```python
from build123d import *

# Parameters (mm, degrees)
EXTRUDE_1_DEPTH      = 13.8
EXTRUDE_1_DEPTH_BACK = 13.8
EXTRUDE_START        = -2
SKETCH_2_W           = 14
SKETCH_2_H           = 6
SKETCH_2_W_2         = 10
SKETCH_2_H_2         = 2
EXTRUDE_2_DEPTH      = 2
EXTRUDE_3_DEPTH      = 1
EXTRUDE_3_DEPTH_BACK = 3
SKETCH_3_R           = 3
EXTRUDE_4_DEPTH      = 3


with BuildPart() as part:
    # Эскиз1 → Бобышка-Вытянуть1 (new, two sides: drawn at the far end of the back side and taken through both)
    with BuildSketch(Plane.XY.offset(-EXTRUDE_1_DEPTH_BACK)):
        with BuildLine():
            Line((-14, 0), (-14.284263959, 1.979695431))
            ThreePointArc((-14.284263959, 1.979695431), (0, 3), (14.284263959, 1.979695431))
            Line((14.284263959, 1.979695431), (14, 0))
            ThreePointArc((14, 0), (0, 1), (-14, 0))
        make_face()
    extrude(amount=EXTRUDE_1_DEPTH + EXTRUDE_1_DEPTH_BACK)

    # Эскиз2 → Бобышка-Вытянуть2 (add)
    with BuildSketch(Plane.XY.offset(13.8).offset(EXTRUDE_START)):
        with Locations((0, -2)):
            Rectangle(SKETCH_2_W, SKETCH_2_H)
        with Locations((0, -2)):
            Rectangle(SKETCH_2_W_2, SKETCH_2_H_2, mode=Mode.SUBTRACT)
    extrude_2 = extrude(amount=-EXTRUDE_2_DEPTH)

    # Зеркальное отражение1: Бобышка-Вытянуть2 across plane
    add(extrude_2.mirror(Plane.XY))

    # Эскиз3 → Бобышка-Вытянуть3 (add, two sides: drawn at the far end of the back side and taken through both)
    with BuildSketch(Plane(origin=(0, 0, 0), x_dir=(1, 0, 0), z_dir=(0, 1, 0)).offset(-EXTRUDE_3_DEPTH_BACK)):
        with Locations(Location((0, 0, 0), (0, 0, 270))):
            Circle(SKETCH_3_R)
    extrude(amount=EXTRUDE_3_DEPTH + EXTRUDE_3_DEPTH_BACK)

    # Эскиз4 → Бобышка-Вытянуть4 (add)
    with BuildSketch(Plane(origin=(0, -3, 0), x_dir=(-1, 0, 0), z_dir=(0, -1, 0))):
        with BuildLine():
            Line((-1.122795001, -0.994651388), (-2.092247595, -2.15))
            ThreePointArc((-2.092247595, -2.15), (-3, 0), (-2.092247595, 2.15))
            Line((-2.092247595, 2.15), (-1.122795001, 0.994651388))
            ThreePointArc((-1.122795001, 0.994651388), (-1.5, 0), (-1.122795001, -0.994651388))
        make_face()
        with BuildLine():
            Line((1.422790871, 0.4750433), (2.908078416, 0.736939569))
            ThreePointArc((2.908078416, 0.736939569), (1.5, 2.598076211), (-0.81583082, 2.886939569))
            Line((-0.81583082, 2.886939569), (-0.29999587, 1.469694689))
            ThreePointArc((-0.29999587, 1.469694689), (0.75, 1.299038106), (1.422790871, 0.4750433))
        make_face()
        with BuildLine():
            Line((-0.29999587, -1.469694689), (-0.81583082, -2.886939569))
            ThreePointArc((-0.81583082, -2.886939569), (1.5, -2.598076211), (2.908078416, -0.736939569))
            Line((2.908078416, -0.736939569), (1.422790871, -0.4750433))
            ThreePointArc((1.422790871, -0.4750433), (0.75, -1.299038106), (-0.29999587, -1.469694689))
        make_face()
    extrude(amount=EXTRUDE_4_DEPTH)


solid = part.part
```
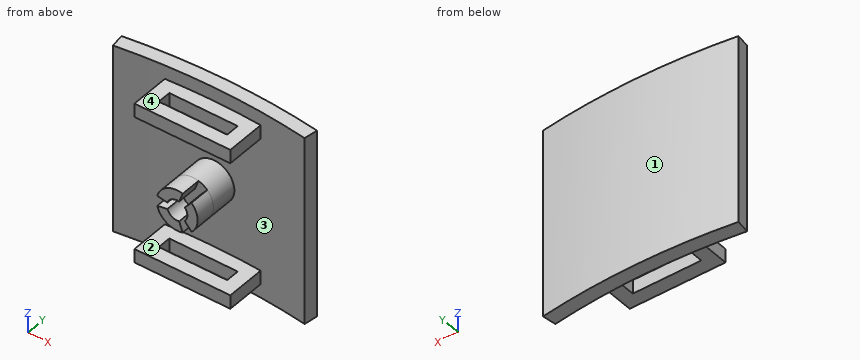
Design review of the part built by this model. Coordinates are the model's own, in mm. Face numbers are marked on the shaded views. Coordinates: 2 decimals unless noted, no trailing zeros. Order: outer loops, then holes, each group sorted by start corner. A loop starts at its lowest first (then second) coordinate and runs counter-clockwise, first axis right, second up. Notation, with made-up numbers: M 36.25,42.5 L 64.25,42.5 A13 ccw 64.25,49.5 Z; hole C 19.5,58.5 d4. An arc over 180 degrees is marked long. Answer as a JSON object with one key per item and string values. Group by question number.
1) For pin 1 (1.6 mm diameter, centred on y = -2, z = -11, fed in from -X); pin 2 (1.6 mm diameter, centred on y = -1.5, z = 11, fed in from +X); pin 3 (1.5 mm diameter, centred on x = -0.5, z = 0.5, fed in from -Y), all flat-tipped, find the tip position at first contact; note any pin that passes through.
2) Add section A-A, the plane y = -4. Write out the cut boundary in (x, z), then the cut area to 3 significant figures.
3) Mouldability with a two-part tool opening along Z and no side actions: class the marked faces 1, 2, 3 and 4 as pulls with the +Z half, pulls with the -Z half, needs draft (parallel to the pull), parting line crosses it, or undercut.
4) Wall thickness on L1, parallel to Z at x = -5.25, y = -1.5; L2, parallel to Z at x = 1.5, y = -0.75; L3, parallel to X at y = -2, z = -10.5: over which ranges is each line inside the solid? List them lowest first.
5) Add section B-B, the plane z = -11. Write out the cut boundary in (x, y), then the cut area to 3 significant figures.
6) Add section D-D, the plane z = -6.5. Write out the cut boundary in (x, y), then the cut area to 3 significant figures.
7) Add section C-C, the plane x = -0.5. Write out the cut boundary in (y, z), then the cut area to 3 significant figures.
Computed values:
{
 "1": {"pin 1": "stops at x = -7", "pin 2": "stops at x = 7", "pin 3": "stops at y = -3"},
 "2": {"outline": "M -7,-11.8 L 7,-11.8 L 7,-9.8 L -7,-9.8 Z; M -7,9.8 L 7,9.8 L 7,11.8 L -7,11.8 Z; M -2.91,-0.74 A3 ccw 0.82,-2.89 L 0.3,-1.47 A1.5 cw -1.42,-0.48 Z; M -2.91,0.74 L -1.42,0.48 A1.5 cw 0.3,1.47 L 0.82,2.89 A3 ccw Z; M 1.12,-0.99 L 2.09,-2.15 A3 ccw 2.09,2.15 L 1.12,0.99 A1.5 cw Z", "area": "71.7 mm^2"},
 "3": {"face 1": "needs draft", "face 2": "undercut", "face 3": "undercut", "face 4": "pulls with the +Z half"},
 "4": {"L1": "z = -11.8 to -9.8, 9.8 to 11.8", "L2": "z = -11.8 to -9.8, -2.6 to 2.6, 9.8 to 11.8", "L3": "x = -7 to -5, 5 to 7"},
 "5": {"outline": "M -14.28,1.98 L -14,0 A98.5 cw -7,0.75 L -7,-5 L 7,-5 L 7,0.75 A98.5 cw 14,0 L 14.28,1.98 A100.5 ccw Z; hole M -5,-3 L 5,-3 L 5,-1 L -5,-1 Z", "area": "120 mm^2"},
 "6": {"outline": "M -14.28,1.98 L -14,0 A98.5 cw 14,0 L 14.28,1.98 A100.5 ccw Z", "area": "56.8 mm^2"},
 "7": {"outline": "M -6,-2.96 L 1,-2.96 L 1,-9.8 L -1,-9.8 L -1,-11.8 L 1,-11.8 L 1,-13.8 L 3,-13.8 L 3,13.8 L 1,13.8 L 1,11.8 L -1,11.8 L -1,9.8 L 1,9.8 L 1,2.96 L -6,2.96 L -6,1.41 L -3,1.41 L -3,-1.41 L -6,-1.41 Z; M -5,-11.8 L -3,-11.8 L -3,-9.8 L -5,-9.8 Z; M -5,9.8 L -3,9.8 L -3,11.8 L -5,11.8 Z", "area": "104 mm^2"}
}
